from build123d import *

# Parameters (mm, degrees)
SKETCH1_R                = 19.45
BOSS_EXTRUDE1_DEPTH      = 6
BOSS_EXTRUDE2_DEPTH      = 10
BOSS_EXTRUDE2_DEPTH_BACK = 6
SKETCH2_R                = 20.5
SKETCH2_R_2              = 19.45


with BuildPart() as part:
    # Sketch1 → Boss-Extrude1 (new body)
    with BuildSketch(Plane(origin=(0, 0, 0), x_dir=(1, 0, 0), z_dir=(0, 1, 0))):
        with Locations(Location((0, 0, 0), (0, 0, 270))):
            Circle(SKETCH1_R)
        with BuildLine():
            Line((1.806258903, -0.5), (-2.363228991, -0.5))
            ThreePointArc((-2.363228991, -0.5), (-2.863228991, 0), (-2.363228991, 0.5))
            Line((-2.363228991, 0.5), (1.806258903, 0.5))
            ThreePointArc((1.806258903, 0.5), (6.25, 0), (1.806258903, -0.5))
        make_face(mode=Mode.SUBTRACT)
    extrude(amount=BOSS_EXTRUDE1_DEPTH)

    # Sketch2 → Boss-Extrude2 (add, two sides: drawn at the far end of the back side and taken through both)
    with BuildSketch(Plane(origin=(0, 6, 0), x_dir=(1, 0, 0), z_dir=(0, 1, 0)).offset(-BOSS_EXTRUDE2_DEPTH_BACK)):
        with Locations(Location((0, 0, 0), (0, 0, 270))):
            Circle(SKETCH2_R)
        with Locations(Location((0, 0, 0), (0, 0, 270))):
            Circle(SKETCH2_R_2, mode=Mode.SUBTRACT)
    extrude(amount=BOSS_EXTRUDE2_DEPTH + BOSS_EXTRUDE2_DEPTH_BACK)


solid = part.part
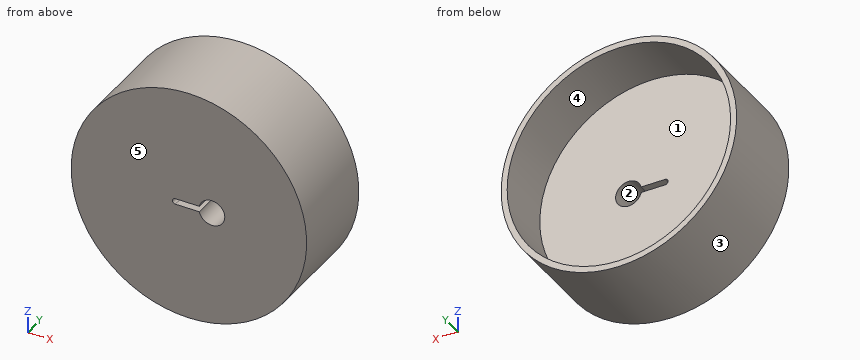
Here's how the part is built. I have some questions about the finished solid (model axes, mm). Face numbers are marked on the shaded views. A direction names the side the tool comes from. Give positions to 0.01 mm unless a question says otherwise; leave off trailing zeros. Loops run counter-clockwise (first coordinate to the right, second up) from the corner with the lowest first, then second, coordinate; pieces in that order, holes last. Notation, with made-up numbers: (-20, 24) -> (18, 24) arc R15 cw to (18, 28) -> close; hole circle Ø2 at (68, -36). An arc over 180 degrees is marked (long way). One line per item, written item: value.
Q1. Suppose I cut it at D-D on x = -10.5. Please give me the cut outline in (y, z).
Answers follow:
outline: (0, -17.61) -> (16, -17.61) -> (16, -16.37) -> (6, -16.37) -> (6, 16.37) -> (16, 16.37) -> (16, 17.61) -> (0, 17.61) -> close
Q2. I'm going to push flat-ended pins straight in: pin 1 Ø5 at (y, z) = (10.5, -16) entering from +X; pin 2 Ø1 at (y, z) = (9.5, 16) entering from -X; pin 3 Ø1 at (x, y) = (14, 14) entering from +Z; pin 4 Ø2.5 at (x, z) = (4, 0) entering from +Y. Where does each tip first touch, or does it pass through?
Answers follow:
pin 1: x = 15.43
pin 2: x = -13.42
pin 3: z = 15.43
pin 4: through
Q3. On a 3-axis mill with a long thin cutter (end or side, diameter ignored), from which of +Z, -Z, +X, -X, +Y, -Y can I reach the whole of each face in a straight line? I mean the marked faces 1 and 2. Say none if no direction works.
Answers follow:
face 1: +Y
face 2: +Y, -Y
Q4. If I drill on line 1 along X through (y, z) = (1.35, 0); line 2 along X through (y, z) = (8.25, 0); line 3 along Y through (x, z) = (-11.5, -12), over which ranges is the centre line in solid material (lowest first)?
Answers follow:
line 1: -20.5 to -2.86, 6.25 to 20.5
line 2: -20.5 to -19.45, 19.45 to 20.5
line 3: 0 to 6
Q5. We'd pull the mould along Z, two halves only. Please class the marked faces 3, 4 and 5: pulls with the +Z half, pulls with the -Z half, needs draft (parallel to the pull), parting line crosses it, or undercut.
Answers follow:
face 3: parting line crosses it
face 4: undercut
face 5: needs draft
Q6. Suppose I cut it at A-A on z = 0. Please give me the cut outline in (x, y), then the cut area to 3 significant figures.
Answers follow:
outline: (-20.5, 0) -> (-2.86, 0) -> (-2.86, 6) -> (-19.45, 6) -> (-19.45, 16) -> (-20.5, 16) -> close; (6.25, 0) -> (20.5, 0) -> (20.5, 16) -> (19.45, 16) -> (19.45, 6) -> (6.25, 6) -> close
area: 212 mm^2
Q7. Suppose I cut it at C-C on y = 14.5. Please give me the cut outline in (x, z), then the cut area to 3 significant figures.
Answers follow:
outline: circle Ø41 at (0, 0); hole circle Ø38.9 at (0, 0)
area: 132 mm^2
Q8. Suppose I cut it at B-B on x = 4. Please give me the cut outline in (y, z).
Answers follow:
outline: (0, -20.11) -> (16, -20.11) -> (16, -19.03) -> (6, -19.03) -> (6, -2.25) -> (0, -2.25) -> close; (0, 2.25) -> (6, 2.25) -> (6, 19.03) -> (16, 19.03) -> (16, 20.11) -> (0, 20.11) -> close
